Part model, mm, in its own coordinate system. A direction names the side the tool comes from. Coordinates: 2 decimals unless noted, no trailing zeros. Order: outer loops, then holes, each group sorted by start corner. A loop starts at its lowest first (then second) coordinate and runs counter-clockwise, first axis right, second up. Notation, with made-up numbers: M 79,5 L 113,5 A16 ccw 113,24 Z; hole C 69.5,-3.5 d1. An arc over 180 degrees is marked long. Write item = value, one per line. Start each with the question number.
from build123d import *

# Parameters (mm, degrees)
F0_R     = 298.45
F0_R_2   = 12.7
F0_R_3   = 216.637975
F1_DEPTH = 6.35
F3_R     = 222.25
F3_R_2   = 215.9
F4_DEPTH = 400.05
F6_R     = 222.25
F6_R_2   = 6.35
F7_DEPTH = 6.35


with BuildPart() as f1:
    # F0 (on Top) → F1 (new body)
    with BuildSketch(Plane.XY):
        Circle(F0_R)
        with Locations((-197.565635, -197.565635)):
            Circle(F0_R_2, mode=Mode.SUBTRACT)
        with Locations((0, -279.4)):
            Circle(F0_R_2, mode=Mode.SUBTRACT)
        with Locations((197.565635, -197.565635)):
            Circle(F0_R_2, mode=Mode.SUBTRACT)
        with Locations((-279.4, 0)):
            Circle(F0_R_2, mode=Mode.SUBTRACT)
        with Locations((-197.565635, 197.565635)):
            Circle(F0_R_2, mode=Mode.SUBTRACT)
        Circle(F0_R_3, mode=Mode.SUBTRACT)
        with Locations((279.4, 0)):
            Circle(F0_R_2, mode=Mode.SUBTRACT)
        with Locations((0, 279.4)):
            Circle(F0_R_2, mode=Mode.SUBTRACT)
        with Locations((197.565635, 197.565635)):
            Circle(F0_R_2, mode=Mode.SUBTRACT)
    extrude(amount=F1_DEPTH)

    # F3 (on offset) → F4 (join)
    with BuildSketch(Plane.XY.offset(6.35)):
        Circle(F3_R)
        Circle(F3_R_2, mode=Mode.SUBTRACT)
    extrude(amount=F4_DEPTH)

    # F6 (on offset) → F7 (join)
    with BuildSketch(Plane.XY.offset(406.4)):
        Circle(F6_R)
        Circle(F6_R_2, mode=Mode.SUBTRACT)
    extrude(amount=F7_DEPTH)


solid = f1.part
Item 1: Cut at D-D, the plane y = 81.5. Write the cut outline in (x, z).
Item 2: Pull direction X, two halves, no side cores. Call faces 4 (the cylindrical face through (-236.84, -181.6, 3.13)), 5 (the flat face through (-3, -46, 412.75)), 6 (the cylindrical face through (-171.916, -131.821, 3.131)): pulls with the +X half, pulls with the -X half, needs draft (parallel to the pull), parting line crosses it, or undercut.
Item 3: 3-axis set-ups, long thin cutter, end or side, ignore diameter. For faces 1 (the cylindrical face through (-292.088, 0.558, 3.131)), 2 (the cylindrical face through (-159.127, 145.915, 203.575)), 3 (the cylindrical face through (-28.93, 220.36, 206.71)): which of +Z, -Z, +X, -X, +Y, -Y reach the whole face in a straight line?
Item 4: Cut at A-A, the plane x = -279.4. Write the cut outline in (y, z).
Item 5: Cut at C-C, the plane z = 237. Write the cut outline in (x, y), and give its area (3 significant figures).
Item 6: Wall check: line 1 along Y through (x, z) = (0, 4); line 2 along Z through (x, y) = (-133, -255.5); line 3 along X through (y, z) = (-79.5, 212.5). Give the ranges that are in metal, low to high. Write a range as [from, to].
Item 7: Flat gauge pins, fed straight in: pin 1 (1 mm diameter, centred on x = -130.5, z = 361.5, fed in from +Y); pin 2 (15 mm diameter, centred on x = -197.57, y = 197.57, fed in from +Z); pin 3 (6 mm diameter, centred on x = -62, y = -172.5, fed in from -Z); pin 4 (8 mm diameter, centred on x = -165.5, y = -233.5, fed in from +Z). Where does each tip first touch, or does it go through?
Filled sheet:
q1.outline = M -287.11,0 L -200.72,0 L -200.72,6.35 L -199.93,6.35 L -199.93,406.4 L 199.93,406.4 L 199.93,6.35 L 200.72,6.35 L 200.72,0 L 287.11,0 L 287.11,6.35 L 206.77,6.35 L 206.77,412.75 L -206.77,412.75 L -206.77,6.35 L -287.11,6.35 Z
q2.face_4 = parting line crosses it
q2.face_5 = needs draft
q2.face_6 = undercut
q3.face_1 = +Z, -Z
q3.face_2 = -Z
q3.face_3 = +Z
q4.outline = M -104.92,0 L -12.7,0 L -12.7,6.35 L -104.92,6.35 Z; M 12.7,0 L 104.92,0 L 104.92,6.35 L 12.7,6.35 Z
q5.outline = C 0,0 d444.5; hole C 0,0 d431.8
q5.area = 8,740 mm2
q6.line_1 = [-298.45, -292.1], [-266.7, -216.64], [216.64, 266.7], [292.1, 298.45]
q6.line_2 = [0, 6.35]
q6.line_3 = [-207.54, -200.73], [200.73, 207.54]
q7.pin_1 = 180.26
q7.pin_2 = through
q7.pin_3 = 406.4
q7.pin_4 = 6.35
